from build123d import *

# Parameters (mm, degrees)
SKETCH1_R           = 4
SKETCH1_R_2         = 2
BOSS_EXTRUDE1_DEPTH = 3
SKETCH1_3_R         = 2
BOSS_EXTRUDE2_DEPTH = 50
SKETCH2_W           = 1.011920828
SKETCH2_H           = 8.527541141
SKETCH2_W_2         = 8.717276296
SKETCH2_H_2         = 1.011920828
CUT_EXTRUDE1_DEPTH  = 1


with BuildPart() as part:
    # Sketch1 → Boss-Extrude1 (new body)
    with BuildSketch(Plane(origin=(0, 0, 0), x_dir=(1, 0, 0), z_dir=(0, 1, 0))):
        Circle(SKETCH1_R)
        Circle(SKETCH1_R_2, mode=Mode.SUBTRACT)
    extrude(amount=BOSS_EXTRUDE1_DEPTH)

    # Sketch1_3 → Boss-Extrude2 (add)
    with BuildSketch(Plane(origin=(0, 0, 0), x_dir=(1, 0, 0), z_dir=(0, 1, 0))):
        Circle(SKETCH1_3_R)
    extrude(amount=BOSS_EXTRUDE2_DEPTH)

    # Sketch2 → Cut-Extrude1 (cut)
    with BuildSketch(Plane(origin=(0, 0, 0), x_dir=(-1, 0, 0), z_dir=(0, -1, 0))):
        with Locations((0.042163368, -0.073785894)):
            Rectangle(SKETCH2_W, SKETCH2_H)
        with Locations((-0.026352105, 0.036892947)):
            Rectangle(SKETCH2_W_2, SKETCH2_H_2)
    extrude(amount=-CUT_EXTRUDE1_DEPTH, mode=Mode.SUBTRACT)


solid = part.part
Build history of the part. All positions in model axes, mm. A direction names the side the tool comes from. Coordinates: 2 decimals unless noted, no trailing zeros. Write each loop counter-clockwise with the first axis right and the second up, starting at its lowest first coordinate (ties: lowest second). Pieces come first, ordered by that corner, then holes.
(1) Cut at B-B on x = 0. List the corners of the cut face in (y, z).
(2) 3-axis set-ups, long thin cutter, end or side, ignore diameter. For faces 1 (the flat face through (-2.2, 0.5, 0.469)), 2 (the flat face through (-2, 3, 1)), 3 (the flat face through (-0.548, 0.5, 2.2)): which of +Z, -Z, +X, -X, +Y, -Y reach the whole face in a straight line?
(3) Pin check, flat tips, straight feed: pin 1 Ø2 at (y, z) = (22.5, 1.5) entering from +X; pin 2 Ø0.8 at (x, y) = (-2, 0.5) entering from -Z; pin 3 Ø0.5 at (x, y) = (-2.5, 0.5) entering from +Z. Stop position of each tip, or through.
(4) Cut at A-A on z = 0. List the corners of the cut face in (x, y), and give its area (3 significant figures).
(5) Cut at C-C on y = 15. List the corners of the cut face in (x, z), and give its area (3 significant figures).
(6) Mould opens along Z. For faces 4 (the cylindrical face through (0, 26, 2)), 5 (the flat face through (0.464, 0.5, 2.2)), 6 (the flat face through (0, 1, 0)), 7 (the flat face through (2.2, 0.5, 0.469)) say: pulls with the +Z half, pulls with the -Z half, needs draft (parallel to the pull), parting line crosses it, or undercut.
(7) Drill centre lines: line 1 (Z direction, x = 0, y = 41.5); line 2 (Y direction, x = -2, z = 0.5); line 3 (Y direction, x = -0.5, z = 0.5). Where is each one in solid material? Low to high.
Working result:
1. outline: (1, -4) - (3, -4) - (3, -2) - (50, -2) - (50, 2) - (3, 2) - (3, 4) - (1, 4) - close
2. face 1: +X, -X, -Y
2. face 2: +Y
2. face 3: +Z, -Z, -Y
3. pin 1: stops at x = 1.94
3. pin 2: stops at z = -3.67
3. pin 3: stops at z = 3.31
4. outline: (-4, 1) - (4, 1) - (4, 3) - (2, 3) - (2, 50) - (-2, 50) - (-2, 3) - (-4, 3) - close
4. area: 204 mm2
5. outline: circle Ø4 at (0, 0)
5. area: 12.6 mm2
6. face 4: parting line crosses it
6. face 5: needs draft
6. face 6: undercut
6. face 7: undercut
7. line 1: z = -2 to 2
7. line 2: y = 0 to 3
7. line 3: y = 1 to 50
